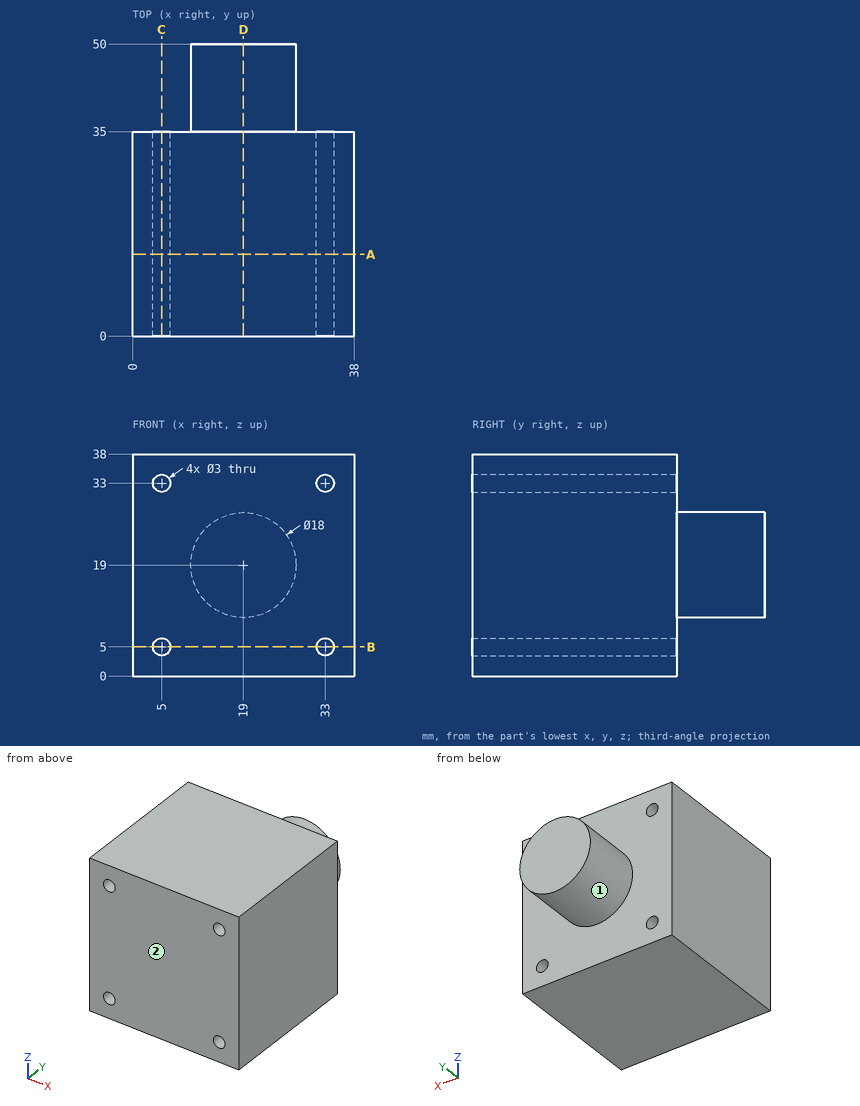
Print and shaded views of the part. All mm, measured from the part's lowest x, y and z. A direction names the side the tool comes from. Coordinates: 2 decimals unless noted, no trailing zeros. Order: outer loops, then holes, each group sorted by start corner. A loop starts at its lowest first (then second) coordinate and runs counter-clockwise, first axis right, second up. Notation, with made-up numbers: (14.25, 81) - (18.25, 81) arc R11 ccw to (18.25, 85) - close; hole circle Ø1 at (67.5, 39.5). An arc over 180 degrees is marked (long way). Return JSON: item names as keys, results as strings. Group by question number.
Item 1: Cut at D-D (x = 19). List the corners of the cut face in (y, z), plus the area to 3 significant figures.
Item 2: Cut at C-C (x = 5). List the corners of the cut face in (y, z).
Item 3: Which spindle directions (+Z, -Z, +X, -X, +Y, -Y) get a long thin tool onto all of the face, cutting with end or side? Do the marked faces 1 and 2. Say none if no direction does.
Item 4: Cut at A-A (y = 14). List the corners of the cut face in (x, z).
Item 5: Drill centre lines: probe 1 along X at (y, z) = (24.5, 5); probe 2 along Z at (x, y) = (33.5, 33). Where is each one in solid material? Low to high. Write a range as from..to.
Item 6: Pin check, flat tips, straight feed: pin 1 (3.5 mm diameter, centred on x = 5, z = 5, fed in from +Y); pin 2 (6 mm diameter, centred on y = 40, z = 12, fed in from -X). Stop position of each tip, or through.
Item 7: Cut at B-B (z = 5). List the corners of the cut face in (x, y), plus the area to 3 significant figures.
Check values:
{
 "1": {"outline": "(0, 0) - (35, 0) - (35, 10) - (50, 10) - (50, 28) - (35, 28) - (35, 38) - (0, 38) - close", "area": "1,600 mm2"},
 "2": {"outline": "(0, 0) - (35, 0) - (35, 3.5) - (0, 3.5) - close; (0, 6.5) - (35, 6.5) - (35, 31.5) - (0, 31.5) - close; (0, 34.5) - (35, 34.5) - (35, 38) - (0, 38) - close"},
 "3": {"face 1": "+Y", "face 2": "+Z, -Z, +X, -X, -Y"},
 "4": {"outline": "(0, 0) - (38, 0) - (38, 38) - (0, 38) - close; hole circle Ø3 at (5, 5); hole circle Ø3 at (5, 33); hole circle Ø3 at (33, 5); hole circle Ø3 at (33, 33)"},
 "5": {"probe 1": "x = 0..3.5, 6.5..31.5, 34.5..38", "probe 2": "z = 0..3.59, 6.41..31.59, 34.41..38"},
 "6": {"pin 1": "stops at y = 35", "pin 2": "stops at x = 10.94"},
 "7": {"outline": "(0, 0) - (3.5, 0) - (3.5, 35) - (0, 35) - close; (6.5, 0) - (31.5, 0) - (31.5, 35) - (6.5, 35) - close; (34.5, 0) - (38, 0) - (38, 35) - (34.5, 35) - close", "area": "1,120 mm2"}
}
